```python
from build123d import *

# Parameters (mm, degrees)
REVOLVE_2_ANGLE     = 90
SHELL_1_T           = -8
SKETCH_3_R          = 4.25
CUT_EXTRUDE_1_DEPTH = 70.282032303
SKETCH_4_R          = 4.25
CUT_EXTRUDE_2_DEPTH = 70.282032303
SKETCH_5_R          = 4.25
CUT_EXTRUDE_3_DEPTH = 70.282032303
CHAMFER_1_SIZE      = 3.55
CHAMFER_2_SIZE      = 3.55
CHAMFER_3_SIZE      = 3.55


with BuildPart() as part:
    # 草图2 → 旋转2 (revolve)
    with BuildSketch(Plane.XY):
        with BuildLine():
            Line((0, 0), (0, 40))
            ThreePointArc((0, 40), (-28.284271247, 28.284271247), (-40, 0))
            Line((-40, 0), (0, 0))
        make_face()
    revolve(axis=Axis((0, 0, 0), (0, 1, 0)), revolution_arc=REVOLVE_2_ANGLE)

    # 抽壳1
    shell_1_openings = [part.faces().sort_by_distance(p)[0] for p in [
        (-20, 28.284271247, 20),
    ]]
    offset(amount=SHELL_1_T, openings=shell_1_openings, kind=Kind.INTERSECTION)

    # 草图3 → 切除-拉伸1 (cut, through all)
    with BuildSketch(Plane(origin=(0, 0, 0), x_dir=(0, 0, -1), z_dir=(1, 0, 0))):
        with Locations((-20, 20)):
            Circle(SKETCH_3_R)
    extrude(amount=-CUT_EXTRUDE_1_DEPTH, mode=Mode.SUBTRACT)

    # 草图4 → 切除-拉伸2 (cut, through all)
    with BuildSketch(Plane(origin=(0, 0, 0), x_dir=(-1, 0, 0), z_dir=(0, 0, -1))):
        with Locations((20, 20)):
            Circle(SKETCH_4_R)
    extrude(amount=-CUT_EXTRUDE_2_DEPTH, mode=Mode.SUBTRACT)

    # 草图5 → 切除-拉伸3 (cut, through all)
    with BuildSketch(Plane.XZ):
        with Locations(Location((-20, 20, 0), (0, 0, 270))):
            Circle(SKETCH_5_R)
    extrude(amount=-CUT_EXTRUDE_3_DEPTH, mode=Mode.SUBTRACT)

    # 倒角1
    chamfer_1_edges = [part.edges().sort_by_distance(p)[0] for p in [
        (-8, 20, 24.25),
    ]]
    chamfer(chamfer_1_edges, length=CHAMFER_1_SIZE)

    # 倒角2
    chamfer_2_edges = [part.edges().sort_by_distance(p)[0] for p in [
        (-15.75, 20, 8),
    ]]
    chamfer(chamfer_2_edges, length=CHAMFER_2_SIZE)

    # 倒角3
    chamfer_3_edges = [part.edges().sort_by_distance(p)[0] for p in [
        (-20, 8, 24.25),
    ]]
    chamfer(chamfer_3_edges, length=CHAMFER_3_SIZE)

    # 草图9 → 切除-旋转2 (revolve, cut)
    with BuildSketch(Plane(origin=(0, 0, 0), x_dir=(-0.7071067811865464, 0, 0.7071067811865488), z_dir=(-0.7071067811865488, 0, -0.7071067811865464)), mode=Mode.PRIVATE) as cut_revolve_2_sk:
        Polygon((-5.259009462, -3.718681253), (16.625182172, 11.755779052), (17.202532441, 10.939282471), (-4.592338975, -4.472018902), align=None)
    revolve(cut_revolve_2_sk.sketch.rotate(Axis((3.718681253, -3.718681253, -3.718681253), (-0.5773502691896244, 0.5773502691896266, 0.5773502691896265)), 180), axis=Axis((3.718681253, -3.718681253, -3.718681253), (-0.5773502691896244, 0.5773502691896266, 0.5773502691896265)), mode=Mode.SUBTRACT)


solid = part.part
```
Input: part model. Units: mm. Frame: model coordinates. A direction names the side the tool comes from. Give positions to 0.01 mm unless a question says otherwise; leave off trailing zeros. Order: outer loops, then holes, each group sorted by start corner. A loop starts at its lowest first (then second) coordinate and runs counter-clockwise, first axis right, second up. Notation, with made-up numbers: M 84.25,74.5 L 96.25,74.5 A26 ccw 96.25,89.5 Z; hole C 14,12 d4. An arc over 180 degrees is marked long. Return JSON: item names as keys, results as strings.
1) Mould query, pull axis Z, two halves, no side actions, for faces 3 (the face through (-27, 27, 8)), 4 (the face through (-4.62, 16.08, 17.96)), 5 (the face through (-8, 27, 27)). Classes: released by +Z, released by -Z, zero draft, split by the parting line, or undercut.
Taken from the geometry:
{"face 3": "released by +Z", "face 4": "undercut", "face 5": "zero draft"}
2) Section query A-A on y = 20. Output: boundary loops of the cut face in (x, z), and give its area (3 significant figures).
Taken from the geometry:
{"outline": "M -34.64,0 L -24.25,0 L -24.25,4.45 L -27.8,8 L -33.7,8 A34.64 ccw Z; M -15.75,0 L 0,0 L 0,15.75 L -4.45,15.75 L -8,12.2 L -8,8 L -12.2,8 L -15.75,4.45 Z; M -8,27.8 L -4.45,24.25 L 0,24.25 L 0,34.64 A34.64 ccw -8,33.7 Z", "area": "324 mm2"}
3) Section query D-D on y = 33. Output: boundary loops of the cut face in (x, z).
Taken from the geometry:
{"outline": "M -22.61,0 L 0,0 L 0,22.61 A22.61 ccw -8,21.14 L -8,8 L -21.14,8 A22.61 ccw Z"}
4) Contact query for flat-ended pins moving along their axis: pin 1 (9 mm diameter, centred on x = -16.5, y = 26.5, fed in from +Z); pin 2 (3 mm diameter, centred on x = -17.5, y = 15.5, fed in from +Z); pin 3 (1.5 mm diameter, centred on y = 12, z = 6.5, fed in from -X). Output: stop coordinate, or through.
Taken from the geometry:
{"pin 1": "stops at z = 8", "pin 2": "stops at z = 6.85", "pin 3": "stops at x = -37.86"}
5) Line query: L1, parallel to Z at x = -26.5, y = 24.5; L2, parallel to X at y = 35, z = 12; L3, parallel to Y at x = -25, z = 6. Output: solid intervals per line, ascending. Write a range as [from, to].
Taken from the geometry:
{"L1": "z = [0, 8]", "L2": "x = [-8, 0]", "L3": "y = [0, 17.06], [22.94, 30.64]"}
6) Access query for faces 1 (the face through (-16, 16, 0)), 2 (the face through (-12.8, 8, 23.4)). Directions: +Z, -Z, +X, -X, +Y, -Y. A direction counts if a zero-diameter tool reaches every point of the face in a straight line with its end or side. Return the directions, or none.
Taken from the geometry:
{"face 1": "-Z, +X, -X, +Y, -Y", "face 2": "+Z, -X, +Y"}
7) Section query C-C on x = -35.5. Output: boundary loops of the cut face in (y, z).
Taken from the geometry:
{"outline": "M 0,0 L 18.43,0 A18.43 ccw 16.61,8 L 8,8 L 8,16.61 A18.43 ccw 0,18.43 Z"}
